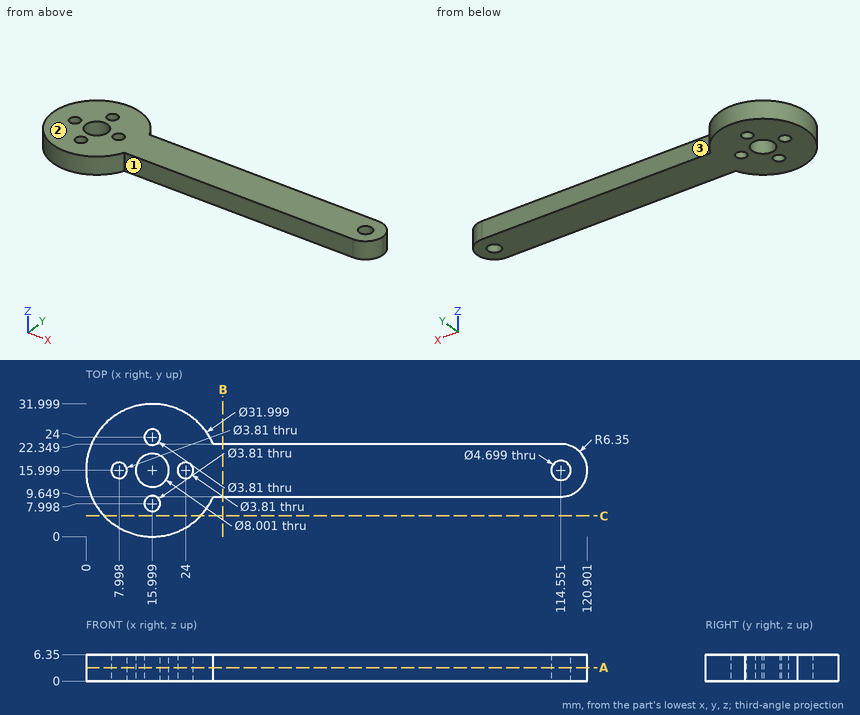
Input: dimensioned drawing with shaded views. Units: mm. Origin: part minimum x, y, z. A direction names the side the tool comes from. Give positions to 0.01 mm unless a question says otherwise; leave off trailing zeros. Loops run counter-clockwise (first coordinate to the right, second up) from the corner with the lowest first, then second, coordinate; pieces in that order, holes last. Notation, with made-up numbers: (-9, 47.25) -> (12, 47.25) arc R7 ccw to (12, 53.25) -> close; hole circle Ø5 at (-17, 5). An arc over 180 degrees is marked (long way). Return JSON: item names as keys, results as strings.
Item 1: Line query: line 1 (X direction, y = 16, z = 3) (1 decimal); line 2 (X direction, y = 14, z = 5.75) (1 decimal); line 3 (X direction, y = 15.5, z = 4.75) (1 decimal). Output: solid intervals per line, ascending.
Filled in:
{"line 1": "0 to 6.1, 9.9 to 12, 20 to 22.1, 25.9 to 112.2, 116.9 to 120.9", "line 2": "0.1 to 12.5, 19.5 to 113.3, 115.8 to 120.6", "line 3": "0 to 6.2, 9.8 to 12, 20 to 22.2, 25.8 to 112.3, 116.8 to 120.9"}
Item 2: Section C-C, the plane y = 5. Output: boundary loops of the cut face in (x, z), plus the area to 3 significant figures.
Filled in:
{"outline": "(4.38, 0) -> (27.62, 0) -> (27.62, 6.35) -> (4.38, 6.35) -> close", "area": "148 mm^2"}
Item 3: Section A-A, the plane z = 3.25. Count the separate pieces of the cut face and the enclosed holes in it, plus the area to 3 significant figures.
Filled in:
{"separate pieces": "1", "enclosed holes": "6", "area": "1,810 mm^2"}
Item 4: Section B-B, the plane x = 33. Output: boundary loops of the cut face in (y, z).
Filled in:
{"outline": "(9.65, 0) -> (22.35, 0) -> (22.35, 6.35) -> (9.65, 6.35) -> close"}
Item 5: Pin query (flat end, axial travel): P1, Ø3, axis at x = 103.5, z = 1.5, coming from the -Y side; P2, Ø3.5, axis at x = 16, y = 24, coming from the +Z side. Return the tip coordinate at first contact, or that it passes through.
Filled in:
{"P1": "y = 9.65", "P2": "through"}
Item 6: Access query for the marked faces 1, 2 and 3. Directions: +Z, -Z, +X, -X, +Y, -Y. A direction counts if a zero-diameter tool reaches every point of the face in a straight line with its end or side. Return the directions, or none.
Filled in:
{"face 1": "+Z, -Z, +X, -Y", "face 2": "+Z, +X, -X, +Y, -Y", "face 3": "+Z, -Z, +X, +Y"}
